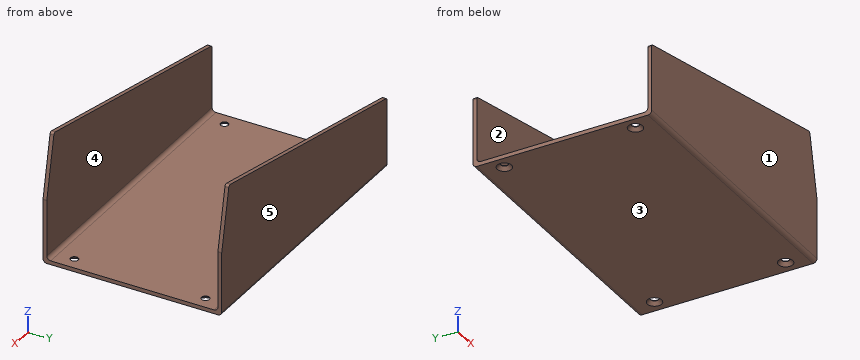
```python
from build123d import *

# Parameters (mm, degrees)
F1_DEPTH       = 37.5
F2_T           = -1.6
F3_R           = 1.6
F5_D           = 3.2
F5_CSINK_D     = 6
F5_CSINK_ANGLE = 90
F6_R           = 1.6
F7_R           = 1


# Not quite as in the source:
# - a feature names something its author has since deleted; it is built from what else it names


with BuildPart() as f1:
    # F0 (on Front) → F1 (new body, symmetric)
    with BuildSketch(Plane.XZ):
        Polygon((-50.4974494928, -20.8124593111), (69.5025505072, -20.8124593111), (69.5025505072, 6.0025406889), (64.2012187523, 32.0403523478), (-50.4975286176, 8.6875406888), align=None)
    extrude(amount=F1_DEPTH, both=True)

    # F2
    f2_openings = [f1.faces().sort_by_distance(p)[0] for p in [
        (-50.497489, 0, -6.062459),
        (6.851845, 0, 20.363947),
        (66.851885, 0, 19.021447),
        (69.502551, 0, -7.404959),
    ]]
    offset(amount=F2_T, openings=f2_openings, kind=Kind.INTERSECTION)

    # F3
    f3_edges = [f1.edges().sort_by_distance(p)[0] for p in [
        (9.502548, -35.9, -19.212459),
        (9.502548, 35.9, -19.212459),
    ]]
    fillet(f3_edges, radius=F3_R)

    # F5 (through all)
    with Locations(Plane(origin=(0, 0, -20.8124593111), x_dir=(1, 0, 0), z_dir=(0, 0, -1))):
        with Locations((64.0025505072, -27.5), (-44.9974494928, -27.5), (64.0025505072, 27.5), (-44.9974494928, 27.5)):
            CounterSinkHole(F5_D / 2, F5_CSINK_D / 2, counter_sink_angle=F5_CSINK_ANGLE)

    # F6
    f6_edges = [f1.edges().sort_by_distance(p)[0] for p in [
        (9.502551, 37.5, -20.812459),
        (9.502551, -37.5, -20.812459),
    ]]
    fillet(f6_edges, radius=F6_R)

    # F7
    f7_edges = [f1.edges().sort_by_distance(p)[0] for p in [
        (64.201219, -36.7, 32.040352),
        (64.201219, 36.7, 32.040352),
        (69.502551, 36.7, 6.002541),
        (69.502551, -36.7, 6.002541),
        (-50.497529, -36.7, 8.687541),
        (-50.497529, 36.7, 8.687541),
    ]]
    fillet(f7_edges, radius=F7_R)


solid = f1.part
```
The listing builds one solid part. Answer for the finished solid, in the listing's coordinates (mm). Face numbers are marked on the shaded views. A direction names the side the tool comes from. Give positions to 0.01 mm unless a question says otherwise; leave off trailing zeros. Order: outer loops, then holes, each group sorted by start corner. A loop starts at its lowest first (then second) coordinate and runs counter-clockwise, first axis right, second up. Notation, with made-up numbers: M -13,82.5 L 37,82.5 A30 cw 37,111.5 Z; hole C -26.5,-39 d6. An arc over 180 degrees is marked long. Put each result on its own line as item: value. Start each with the question number.
Item 1: Flat-ended cylindrical pins translate along their axes: P1, Ø12, axis at x = 45.5, y = -13.5, coming from the +Z side; P2, Ø4, axis at x = 64, y = 27.5, coming from the -Z side (3 decimals); P3, Ø5, axis at x = -45, y = 27.5, coming from the -Z side (3 decimals). Find the tip coordinate at first contact, or state that the pin passes through.
Item 2: Which of the six approach directions +Z, -Z, +X, -X, +Y, -Y give full straight-line access (tool end or side, diameter ignored) to the marked faces 4 and 5?
Item 3: Find the intervals of material crossed by line 1 along X through (y, z) = (-27.5, -19.25); line 2 along Y through (x, z) = (-5.5, -10.5); line 3 along Z through (x, y) = (40.5, -1), in increasing order.
Item 4: For a pull along Y with two mould halves and no side action, classify the marked faces 1, 2 and 3 as +Y half, -Y half, draft (parallel to the pull), parting line (faces both ways), or undercut.
Item 5: The part is cut by section C-C, the plane x = 12. Determine the outline of the cut face in (y, z), and give its area (3 significant figures).
Item 6: The part is cut by section A-A, the plane y = -27.5. Determine the outline of the cut face in (x, z), and give its area (3 significant figures).
Item 7: The part is cut by section D-D, the plane z = -11.5. Determine the outline of the cut face in (x, y).
Item 8: The part is cut by section B-B, the plane z = 10.5. Determine the outline of the cut face in (x, y), and give its area (3 significant figures).
Answer key:
1. P1: stops at z = -19.21
1. P2: stops at z = -19.815
1. P3: stops at z = -20.315
2. face 4: +Z, +X, -X
2. face 5: +Z, -Z, +X, -X, +Y
3. line 1: x = -50.5 to -46.6, -43.4 to 62.4, 65.6 to 69.5
3. line 2: y = -37.5 to -35.9, 35.9 to 37.5
3. line 3: z = -20.81 to -19.21
4. face 1: -Y half
4. face 2: undercut
4. face 3: draft
5. outline: M -37.5,-19.21 A1.6 ccw -35.9,-20.81 L 35.9,-20.81 A1.6 ccw 37.5,-19.21 L 37.5,21.41 L 35.9,21.41 L 35.9,-17.61 A1.6 cw 34.3,-19.21 L -34.3,-19.21 A1.6 cw -35.9,-17.61 L -35.9,21.41 L -37.5,21.41 Z
5. area: 250 mm²
6. outline: M -50.5,-20.81 L -48,-20.81 L -46.6,-19.41 L -46.6,-19.21 L -50.5,-19.21 Z; M -43.4,-19.41 L -42,-20.81 L 61,-20.81 L 62.4,-19.41 L 62.4,-19.21 L -43.4,-19.21 Z; M 65.6,-19.41 L 67,-20.81 L 69.5,-20.81 L 69.5,-19.21 L 65.6,-19.21 Z
6. area: 178 mm²
7. outline: M -50.5,-37.5 L 69.5,-37.5 L 69.5,-35.9 L -50.5,-35.9 Z; M -50.5,35.9 L 69.5,35.9 L 69.5,37.5 L -50.5,37.5 Z
8. outline: M -41.6,-37.5 L 68.59,-37.5 L 68.59,-35.9 L -41.6,-35.9 Z; M -41.6,35.9 L 68.59,35.9 L 68.59,37.5 L -41.6,37.5 Z
8. area: 353 mm²
